Geometry: final body of the model. Coordinates: model frame, mm. A direction names the side the tool comes from. Give positions to 0.01 mm unless a question says otherwise; leave off trailing zeros. Write each loop counter-clockwise with the first axis right and the second up, starting at its lowest first coordinate (ties: lowest second). Pieces come first, ordered by that corner, then holes. Notation, with made-up numbers: M -36.5,64 L -7.5,64 A25 ccw -7.5,100 Z; hole C 19.25,-17 d9. An arc over 180 degrees is marked long. Use a Markdown table: item, result. Add a question column.
(1) Cut plane B-B (z = -1.5). Output: boundary loops of the cut face in (x, y).
(2) Material intervals for L1, parallel to X at y = 2.5, z = -3.5; L2, parallel to X at y = 4, z = 16; L3, parallel to Y at x = -0.5, z = -13, sorted ascending.
(3) Reachability of faces 1 (the flat face through (-6, -2, 10.16)), 2 (the conical face through (3.1, -5.9, 19.7)) from +Z, -Z, +X, -X, +Y, -Y: full face, straight path, thin tool, end or side. Return the list, or none.
(4) Pin query (flat end, axial travel): pin 1 Ø5 at (y, z) = (5, 6) entering from -X; pin 2 Ø2 at (x, z) = (2, -4) entering from -Y; pin 3 Ø1.5 at (x, z) = (5, 19.5) entering from +Y. Return the tip coordinate at first contact, or that it passes through.
(5) Cut plane A-A (z = 6). Output: boundary loops of the cut face in (x, y).
```python
from build123d import *

# Parameters (mm, degrees)
F0_R     = 5.74675
F1_DEPTH = 10.16
F2_R     = 8.1915
F2_R_2   = 5.74675
F3_DEPTH = 1.905
F4_R     = 8.1915
F5_DEPTH = 12.7
F6_SIZE2 = 12.7
F6_SIZE  = 2.54
F7_DEPTH = 17.272
F8_SIZE2 = 5.74039
F8_SIZE  = 17.27199


# Not quite as in the source:
# - a fillet or chamfer is up to 0.001 mm smaller than in the source, because OpenCascade refuses the exact size


with BuildPart() as f1:
    # F0 (on Top) → F1 (new body)
    with BuildSketch(Plane.XY):
        Circle(F0_R)
    extrude(amount=F1_DEPTH)

    # F2 (on face) → F3 (join)
    with BuildSketch(Plane.XY.offset(10.16)):
        Circle(F2_R)
        Circle(F2_R_2, mode=Mode.SUBTRACT)
        Circle(F2_R_2)
    extrude(amount=F3_DEPTH)

    # F4 (on face) → F5 (join)
    with BuildSketch(Plane.XY.offset(12.065)):
        Circle(F4_R)
    extrude(amount=F5_DEPTH)

    # F6
    f6_edges = [f1.edges().sort_by_distance(p)[0] for p in [
        (-8.1915, 0, 24.765),
    ]]
    f6_side = f1.faces().sort_by_distance((0, 0, 24.765))[0]
    chamfer(f6_edges, length=F6_SIZE, length2=F6_SIZE2, reference=f6_side)

    # F7 (add): a face of the model
    f7_faces = [f1.faces().sort_by_distance(p)[0] for p in [
        (0, 0, 0),
    ]]
    extrude(f7_faces, amount=F7_DEPTH)

    # F8 (size 17.272 and 5.7404 in the source; OpenCascade refuses exactly that, so slightly less here)
    f8_edges = [f1.edges().sort_by_distance(p)[0] for p in [
        (-5.74675, 0, -17.272),
    ]]
    f8_side = f1.faces().sort_by_distance((-5.74675, 0, -8.636))[0]
    chamfer(f8_edges, length=F8_SIZE, length2=F8_SIZE2, reference=f8_side)


solid = f1.part
```
Answer list:
| question | item | result |
|---|---|---|
| 1 | outline | C 0,0 d10.5 |
| 2 | L1 | -3.84 to 3.84 |
| 2 | L2 | -6.23 to 6.23 |
| 2 | L3 | -1.34 to 1.34 |
| 3 | face 1 | -Z |
| 3 | face 2 | +Z |
| 4 | pin 1 | x = -5.17 |
| 4 | pin 2 | y = -4.47 |
| 4 | pin 3 | y = 5.22 |
| 5 | outline | C 0,0 d11.49 |
